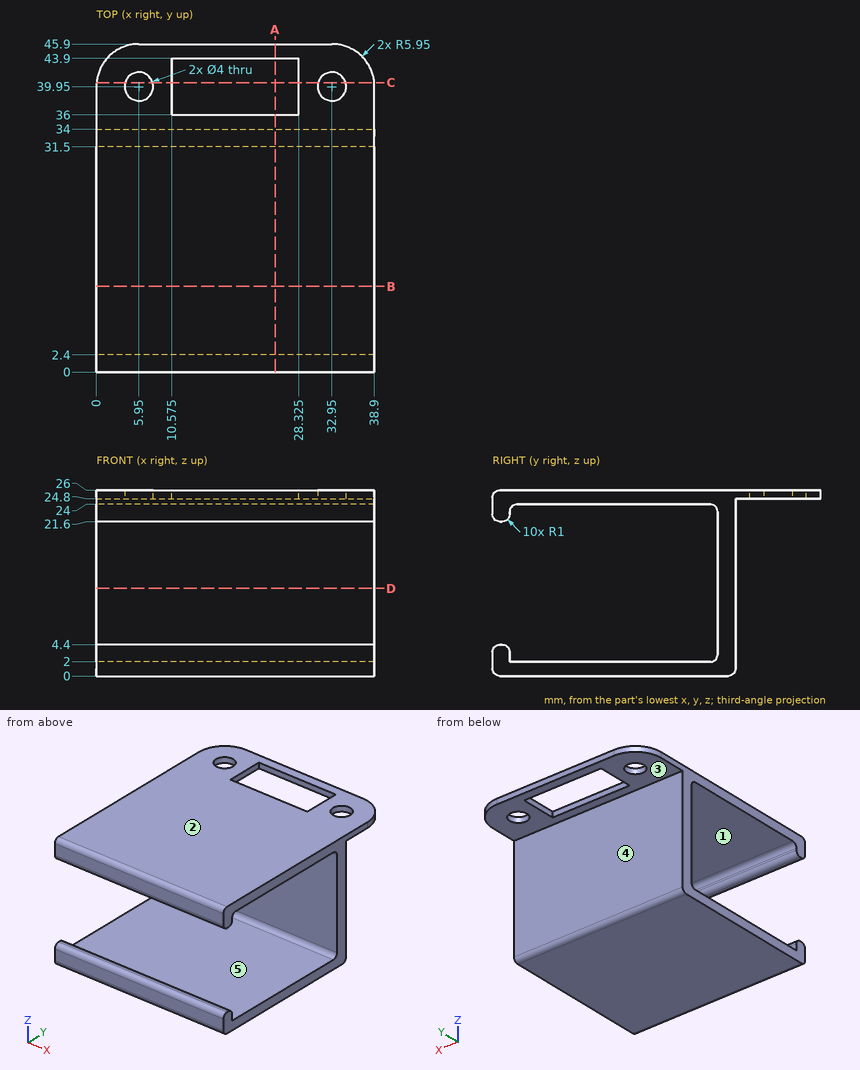
The figure shows three views and two pictorial views of one solid part (mm, origin at its lowest corner). Answer the questions. A direction names the side the tool comes from. Coordinates: 2 decimals unless noted, no trailing zeros. Loops run counter-clockwise (first coordinate to the right, second up) from the corner with the lowest first, then second, coordinate; pieces in that order, holes last.
1) Find the intervals of material crossed by L1, parallel to Z at x = 33, y = 15.5; L2, parallel to Y at x = 5.95, z = 25.5; L3, parallel to Y at x = 19, z = 15, in increasing order.
2) Flat-ended cylindrical pins translate along their axes: pin 1 Ø4.5 at (x, y) = (32.95, 39.95) entering from +Z; pin 2 Ø3 at (x, z) = (33, 8.5) entering from -Y; pin 3 Ø6 at (x, y) = (23.5, 42.5) entering from -Z; pin 4 Ø0.6 at (y, z) = (41.5, 25.5) entering from +X. Find the tip coordinate at first contact, or state that the pin passes through.
3) Find section B-B on y = 12. Write down the section's boundary in (x, z).
4) Find section A-A on x = 25. Write down the section's boundary in (y, z).
5) Determine the mould class of the marked faces 3, 4 and 5 for opening direction Y: pulls with the +Y half, pulls with the -Y half, needs draft (parallel to the pull), parting line crosses it, or undercut.
6) Find section C-C on y = 40.5. Write down the section's boundary in (x, z) (3 decimals).
7) Find section D-D on z = 12.25. Write down the section's boundary in (x, y), then the cut area to 4 significant figures.
8) A tool of negligible diameter and unlimited length cuts with its end or side. For the marked faces 1 and 2, from which of +Z, -Z, +X, -X, +Y, -Y can it reach the whole face along a straight path? Write none if from no direction.
Values:
1. L1: z = 0 to 2, 24 to 26
1. L2: y = 0.13 to 37.95, 41.95 to 45.9
1. L3: y = 31.5 to 34
2. pin 1: stops at z = 26
2. pin 2: stops at y = 31.5
2. pin 3: stops at z = 24.8
2. pin 4: stops at x = 38.77
3. outline: (0, 0) - (38.9, 0) - (38.9, 2) - (0, 2) - close; (0, 24) - (38.9, 24) - (38.9, 26) - (0, 26) - close
4. outline: (0, 1) arc R1 ccw to (1, 0) - (33, 0) arc R1 ccw to (34, 1) - (34, 24.8) - (36, 24.8) - (36, 26) - (1, 26) arc R1 ccw to (0, 25) - (0, 22.6) arc R1 ccw to (1, 21.6) - (1.4, 21.6) arc R1 ccw to (2.4, 22.6) - (2.4, 23) arc R1 cw to (3.4, 24) - (30.5, 24) arc R1 cw to (31.5, 23) - (31.5, 3) arc R1 cw to (30.5, 2) - (2.4, 2) - (2.4, 3.4) arc R1 ccw to (1.4, 4.4) - (1, 4.4) arc R1 ccw to (0, 3.4) - close; (43.9, 24.8) - (45.9, 24.8) - (45.9, 26) - (43.9, 26) - close
5. face 3: needs draft
5. face 4: pulls with the +Y half
5. face 5: undercut
6. outline: (0.025, 24.8) - (4.027, 24.8) - (4.027, 26) - (0.025, 26) - close; (7.873, 24.8) - (10.575, 24.8) - (10.575, 26) - (7.873, 26) - close; (28.325, 24.8) - (31.027, 24.8) - (31.027, 26) - (28.325, 26) - close; (34.873, 24.8) - (38.875, 24.8) - (38.875, 26) - (34.873, 26) - close
7. outline: (0, 31.5) - (38.9, 31.5) - (38.9, 34) - (0, 34) - close
7. area: 97.25 mm2
8. face 1: +X, -X
8. face 2: +Z, +X, -X, +Y, -Y
